Could you check a few things on this model? Use its own coordinates, in mm. A direction names the side the tool comes from. Give positions to 0.01 mm unless a question says otherwise; leave off trailing zeros. Write each loop counter-clockwise with the first axis right and the second up, starting at its lowest first coordinate (ties: lowest second). Pieces come first, ordered by that corner, then holes. Notation, with made-up numbers: (-26, -40) - (3, -40) arc R25 cw to (3, -25) - close; hole circle Ø3 at (23.25, 39.5). An arc over 180 degrees is marked (long way). Answer as a JSON object with one key per item and string values. Group by question number.
```python
from build123d import *

# Parameters (mm, degrees)
SKETCH_1_W               = 40
SKETCH_1_H               = 41
EXTRUDE_1_DEPTH          = 2
FILLET_1_R               = 3
SKETCH_2_R               = 1.6
CUT_EXTRUDE_1_DEPTH      = 50
EXTRUDE_2_DEPTH          = 2
CUT_EXTRUDE_2_DEPTH      = 50
SKETCH_5_R               = 1.6
CUT_EXTRUDE_3_DEPTH      = 50
PATTERN_CIRCULAR_1_COUNT = 6
FILLET_2_R               = 1
FILLET_3_R               = 1


with BuildPart() as part:
    # 草图1 → 凸台-拉伸1 (new body)
    with BuildSketch(Plane(origin=(0, 0, 0), x_dir=(1, 0, 0), z_dir=(0, 1, 0))):
        Rectangle(SKETCH_1_W, SKETCH_1_H)
    extrude(amount=EXTRUDE_1_DEPTH)

    # 圆角1
    fillet_1_edges = [part.edges().sort_by_distance(p)[0] for p in [
        (20, 1, 20.5),
        (-20, 1, 20.5),
    ]]
    fillet(fillet_1_edges, radius=FILLET_1_R)

    # 草图2 → 切除-拉伸1 (cut)
    with BuildSketch(Plane(origin=(0, 2, 0), x_dir=(1, 0, 0), z_dir=(0, 1, 0))):
        with Locations(Location((-15, -12.5, 0), (0, 0, 270))):
            Circle(SKETCH_2_R)
        with Locations(Location((-15, 11.5, 0), (0, 0, 270))):
            Circle(SKETCH_2_R)
        with Locations(Location((15, 11.5, 0), (0, 0, 270))):
            Circle(SKETCH_2_R)
        with Locations(Location((15, -12.5, 0), (0, 0, 270))):
            Circle(SKETCH_2_R)
    extrude(amount=-CUT_EXTRUDE_1_DEPTH, mode=Mode.SUBTRACT)

    # 草图3 → 凸台-拉伸2 (add)
    with BuildSketch(Plane(origin=(0, 0, -20.5), x_dir=(-1, 0, 0), z_dir=(0, 0, -1))):
        with BuildLine():
            Line((-20, 0), (20, 0))
            Line((20, 0), (20, 26.5))
            ThreePointArc((20, 26.5), (0, 46.5), (-20, 26.5))
            Line((-20, 26.5), (-20, 0))
        make_face()
    extrude(amount=-EXTRUDE_2_DEPTH)

    # 草图4 → 切除-拉伸2 (cut)
    with BuildSketch(Plane(origin=(0, 0, -20.5), x_dir=(-1, 0, 0), z_dir=(0, 0, -1))):
        with BuildLine():
            Line((6.5, 33.5), (6.5, 19.5))
            ThreePointArc((6.5, 19.5), (0, 13), (-6.5, 19.5))
            Line((-6.5, 19.5), (-6.5, 33.5))
            ThreePointArc((-6.5, 33.5), (0, 40), (6.5, 33.5))
        make_face()
    extrude(amount=-CUT_EXTRUDE_2_DEPTH, mode=Mode.SUBTRACT)

    # 草图5 → 切除-拉伸3 (cut)
    with BuildSketch(Plane(origin=(0, 0, -20.5), x_dir=(-1, 0, 0), z_dir=(0, 0, -1))):
        with Locations((15.5, 26.5)):
            Circle(SKETCH_5_R)
    cut_extrude_3 = extrude(amount=-CUT_EXTRUDE_3_DEPTH, mode=Mode.SUBTRACT)

    # 阵列(圆周)1: 切除-拉伸3 ×6 about axis
    pattern_circular_1_axis = Axis((0, 26.5, 0), (0, 0, 1))
    for i in range(1, PATTERN_CIRCULAR_1_COUNT):
        add(cut_extrude_3.rotate(pattern_circular_1_axis, i * 360 / PATTERN_CIRCULAR_1_COUNT), mode=Mode.SUBTRACT)

    # 圆角2
    fillet_2_edges = [part.edges().sort_by_distance(p)[0] for p in [
        (0, 0, -20.5),
    ]]
    fillet(fillet_2_edges, radius=FILLET_2_R)

    # 圆角3
    fillet_3_edges = [part.edges().sort_by_distance(p)[0] for p in [
        (0, 2, -18.5),
    ]]
    fillet(fillet_3_edges, radius=FILLET_3_R)


solid = part.part
```
(1) If we mould it in two halves opening along Z, with no side actions, what happens to faces 1 (the flat face through (6.5, 26, -20)), 2 (the cylindrical face through (15.07, 1.01, 10.9)), 3 (the cylindrical face through (-19.14, 1.01, 19.6))? For each: +Z half, -Z half, draft (parallel to the pull), parting line (faces both ways), or undercut.
(2) I need wall thicknesses on L1, parallel to X at y = 0.7, z = -11.5; L2, parallel to Z at x = 14.5, y = 7.5; L3, parallel to Y at x = -17, z = -2. Which ranges of each line are inside material? Lowest first, please.
(3) I want a section at A-A, the plane x = 0. Please give me the cut outline in (y, z), and give its area (3 significant figures).
(4) For faces 4 (the flat face through (-9, 20, -18.5)), 5 (the flat face through (-6.5, 27, -20)), 6 (the flat face through (20, 1, -7)), which set-ups out of +Z, -Z, +X, -X, +Y, -Y let a thin tool reach every point of the face, with its end or its side?
(5) I want a section at D-D, the plane x = -15. Please give me the cut outline in (y, z), and give its area (3 significant figures).
(6) I want a section at B-B, the plane z = 12.5. Please give me the cut outline in (x, y).
(7) Will these pins go through, and if not, where does the flat tip stop? P1, Ø1.9, axis at x = -15, z = 12.5, coming from the -Y side; P2, Ø3.5, axis at x = 15.5, y = 26.5, coming from the -Z side; P3, Ø20, axis at x = 2.5, y = 25.5, coming from the +Z side; P4, Ø0.6, axis at y = 27, z = -19, coming from the -X side.
(8) I want a section at C-C, the plane y = 25.5. Please give me the cut outline in (x, z), and give its area (3 significant figures).
Entries:
{
 "1": {"face 1": "draft", "face 2": "undercut", "face 3": "+Z half"},
 "2": {"L1": "-20 to -16.6, -13.4 to 13.4, 16.6 to 20", "L2": "-20.5 to -18.5", "L3": "0 to 2"},
 "3": {"outline": "(0, -19.5) arc R1 ccw to (1, -20.5) - (13, -20.5) - (13, -18.5) - (3, -18.5) arc R1 cw to (2, -17.5) - (2, 20.5) - (0, 20.5) - close; (40, -20.5) - (46.5, -20.5) - (46.5, -18.5) - (40, -18.5) - close", "area": "117 mm^2"},
 "4": {"face 4": "+Z, +X, -X, +Y", "face 5": "+Z, -Z", "face 6": "+Z, -Z, +X, +Y, -Y"},
 "5": {"outline": "(0, -19.5) arc R1 ccw to (1, -20.5) - (24.98, -20.5) - (24.98, -18.5) - (3, -18.5) arc R1 cw to (2, -17.5) - (2, -13.1) - (0, -13.1) - close; (0, -9.9) - (2, -9.9) - (2, 10.9) - (0, 10.9) - close; (0, 14.1) - (2, 14.1) - (2, 20.5) - (0, 20.5) - close; (28.02, -20.5) - (39.73, -20.5) - (39.73, -18.5) - (28.02, -18.5) - close", "area": "139 mm^2"},
 "6": {"outline": "(-20, 0) - (-16.6, 0) - (-16.6, 2) - (-20, 2) - close; (-13.4, 0) - (13.4, 0) - (13.4, 2) - (-13.4, 2) - close; (16.6, 0) - (20, 0) - (20, 2) - (16.6, 2) - close"},
 "7": {"P1": "through", "P2": "z = -20.5", "P3": "z = -18.5", "P4": "x = -20"},
 "8": {"outline": "(-20, -20.5) - (-16.75, -20.5) - (-16.75, -18.5) - (-20, -18.5) - close; (-14.25, -20.5) - (-6.5, -20.5) - (-6.5, -18.5) - (-14.25, -18.5) - close; (6.5, -20.5) - (14.25, -20.5) - (14.25, -18.5) - (6.5, -18.5) - close; (16.75, -20.5) - (20, -20.5) - (20, -18.5) - (16.75, -18.5) - close", "area": "44.0 mm^2"}
}
